```python
from build123d import *

# Parameters (mm, degrees)
SKETCH_1_W          = 22
SKETCH_1_H          = 10
SKETCH_1_R          = 1.25
SKETCH_1_R_2        = 3
EXTRUDE_1_DEPTH     = 9
SKETCH_2_R          = 1.5
CUT_EXTRUDE_1_DEPTH = 11
SKETCH_4_W          = 7
SKETCH_4_H          = 3
CUT_EXTRUDE_2_DEPTH = 10
FILLET_1_R          = 1


with BuildPart() as part:
    # 草图1 → 凸台-拉伸1 (new body)
    with BuildSketch(Plane.XY):
        Rectangle(SKETCH_1_W, SKETCH_1_H)
        with Locations((8, 0)):
            Circle(SKETCH_1_R, mode=Mode.SUBTRACT)
        with Locations(Location((-8, 0, 0), (0, 0, 180))):
            Circle(SKETCH_1_R, mode=Mode.SUBTRACT)
        Circle(SKETCH_1_R_2, mode=Mode.SUBTRACT)
    extrude(amount=EXTRUDE_1_DEPTH)

    # 草图2 → 切除-拉伸1 (cut)
    with BuildSketch(Plane.XZ.offset(5)):
        with Locations(Location((0, 3, 0), (0, 0, 270))):
            Circle(SKETCH_2_R)
    extrude(amount=-CUT_EXTRUDE_1_DEPTH, mode=Mode.SUBTRACT)

    # 草图4 → 切除-拉伸2 (cut)
    with BuildSketch(Plane.XZ.offset(5)):
        with Locations((-7.5, 1.5)):
            Rectangle(SKETCH_4_W, SKETCH_4_H)
        with Locations((7.5, 1.5)):
            Rectangle(SKETCH_4_W, SKETCH_4_H)
    extrude(amount=-CUT_EXTRUDE_2_DEPTH, mode=Mode.SUBTRACT)

    # 圆角1
    fillet_1_edges = [part.edges().sort_by_distance(p)[0] for p in [
        (-4, 5, 1.5),
        (-4, -5, 1.5),
        (4, 5, 1.5),
        (4, -5, 1.5),
        (11, -5, 6),
        (-11, -5, 6),
        (-11, 5, 6),
        (11, 5, 6),
    ]]
    fillet(fillet_1_edges, radius=FILLET_1_R)


solid = part.part
```
Input: part model. Units: mm. Frame: model coordinates. A direction names the side the tool comes from. Coordinates: 2 decimals unless noted, no trailing zeros. Write each loop counter-clockwise with the first axis right and the second up, starting at its lowest first coordinate (ties: lowest second). Pieces come first, ordered by that corner, then holes. Notation, with made-up numbers: M -6.75,8 L 48.25,8 A23 ccw 48.25,45 Z; hole C 44.25,-5.75 d11. An arc over 180 degrees is marked long. Use one line per item in the form item = value.
Q1. Draft query along X for faces 1 (the face through (0, -5, 5)), 2 (the face through (11, 0, 6)), 3 (the face through (-0.575, 3.782, 1.614)). Return one class per face: released by +X, released by -X, zero draft, split by the parting line, or undercut.
Answer below:
face_1 = zero draft
face_2 = released by +X
face_3 = undercut
Q2. Material intervals for probe 1 along Y at (x, z) = (0, 7.25); probe 2 along X at (y, z) = (0.25, 7.5); probe 3 along Z at (x, y) = (0, -3.6), sorted ascending. Write a range as from..to.
Answer below:
probe_1 = -5..-3, 3..5
probe_2 = -11..-9.22, -6.78..-2.99, 2.99..6.78, 9.22..11
probe_3 = 0..1.5, 4.5..9
Q3. Set-up query: faces 4 (the face through (-3.699, -4.715, 1.521)), 5 (the face through (3.699, -4.715, 1.521)), 6 (the face through (2.3, 2.3, 9)), 7 (the face through (4, 0, 1)), 8 (the face through (-3.699, 4.715, 1.521)). Return all of +Z, -Z, +X, -X, +Y, -Y with unobstructed straight access to the full face (end or side cutting, diameter ignored); none if empty.
Answer below:
face_4 = -Z, -X, -Y
face_5 = -Z, +X, -Y
face_6 = +Z, +X, -X, +Y, -Y
face_7 = -Z, +X, +Y, -Y
face_8 = -Z, -X, +Y
Q4. First-contact query: pin 1 (3 mm diameter, centred on x = -4.5, y = 4, fed in from -Z); pin 2 (1.5 mm diameter, centred on y = -0.5, z = 1.5, fed in from -X); pin 3 (2.5 mm diameter, centred on y = 0.5, z = 1.5, fed in from +X). Flat tips, straight axial feed; report the tip coordinate or a pass-through.
Answer below:
pin_1 = 0
pin_2 = -4
pin_3 = 4
Q5. Section C-C (x = 0). Return loops of the section in (y, z).
Answer below:
outline = M -5,0 L -3,0 L -3,1.5 L -5,1.5 Z; M -5,4.5 L -3,4.5 L -3,9 L -5,9 Z; M 3,0 L 5,0 L 5,1.5 L 3,1.5 Z; M 3,4.5 L 5,4.5 L 5,9 L 3,9 Z
Q6. Section B-B (x = 8). Return loops of the section in (y, z).
Answer below:
outline = M -5,3 L -1.25,3 L -1.25,9 L -5,9 Z; M 1.25,3 L 5,3 L 5,9 L 1.25,9 Z
Q7. Section D-D (z = 2.75). Return loops of the section in (x, y), plus the area to 3 significant figures.
Answer below:
outline = M -4,-4 A1 ccw -3,-5 L -1.48,-5 L -1.48,-2.61 A3 cw -1.48,2.61 L -1.48,5 L -3,5 A1 ccw -4,4 Z; M 1.48,-5 L 3,-5 A1 ccw 4,-4 L 4,4 A1 ccw 3,5 L 1.48,5 L 1.48,2.61 A3 cw 1.48,-2.61 Z
area = 38.3 mm²
Q8. Section A-A (y = 0). Return loops of the section in (x, z), plus the area to 3 significant figures.
Answer below:
outline = M -11,3 L -9.25,3 L -9.25,9 L -11,9 Z; M -6.75,3 L -4,3 L -4,0 L -3,0 L -3,9 L -6.75,9 Z; M 3,0 L 4,0 L 4,3 L 6.75,3 L 6.75,9 L 3,9 Z; M 9.25,3 L 11,3 L 11,9 L 9.25,9 Z
area = 72.0 mm²
